Design review of the part built by this model. Coordinates are the model's own, in mm. A direction names the side the tool comes from. Give positions to 0.01 mm unless a question says otherwise; leave off trailing zeros. Write each loop counter-clockwise with the first axis right and the second up, starting at its lowest first coordinate (ties: lowest second). Pieces come first, ordered by that corner, then holes. Notation, with made-up numbers: (-34, 26) -> (3, 26) arc R32 ccw to (3, 63) -> close; hole circle Ø1 at (31, -17). An arc over 180 degrees is marked (long way). Answer as a JSON object with one key per item and string values.
```python
from build123d import *

# Parameters (mm, degrees)
F0_W     = 249.8
F0_H     = 100
F1_DEPTH = 4
F2_W     = 20
F2_H     = 10
F3_DEPTH = 25
F4_W     = 76
F4_H     = 40
F4_W_2   = 48
F4_H_2   = 65
F5_DEPTH = 25
F6_W     = 3.2
F6_H     = 20
F7_DEPTH = 13
F8_SIZE  = 12.1
F9_R     = 1


with BuildPart() as f1:
    # F0 (on Front) → F1 (new body)
    with BuildSketch(Plane.XZ):
        with Locations((45.308904, 9.584513)):
            Rectangle(F0_W, F0_H)
    extrude(amount=F1_DEPTH)

    # F2 (on face) → F3 (cut)
    with BuildSketch(Plane.XZ.offset(4)):
        with Locations((160.208904, -35.415487)):
            Rectangle(F2_W, F2_H)
        with Locations((-69.591096, -35.415487)):
            Rectangle(F2_W, F2_H)
    extrude(amount=-F3_DEPTH, mode=Mode.SUBTRACT)

    # F4 (on face) → F5 (cut)
    with BuildSketch(Plane.XZ.offset(4)):
        with Locations((45.308904, 21.584513)):
            Rectangle(F4_W, F4_H)
        with Locations((-55.591096, 27.084513)):
            Rectangle(F4_W_2, F4_H_2)
        with Locations((146.208904, 27.084513)):
            Rectangle(F4_W_2, F4_H_2)
    extrude(amount=-F5_DEPTH, mode=Mode.SUBTRACT)

    # F6 (on face) → F7 (join)
    with BuildSketch(Plane(origin=(0, 0, 0), x_dir=(-1, 0, 0), z_dir=(0, 1, 0))):
        with Locations((-123.808904, -17.415487)):
            Rectangle(F6_W, F6_H)
    extrude(amount=F7_DEPTH)

    # F8
    f8_edges = [f1.edges().sort_by_distance(p)[0] for p in [
        (123.808904, 13, -7.415487),
    ]]
    chamfer(f8_edges, length=F8_SIZE)

    # F9
    f9_edges = [f1.edges().sort_by_distance(p)[0] for p in [
        (123.808904, 13, -27.415487),
    ]]
    fillet(f9_edges, radius=F9_R)


solid = f1.part
```
(1) We need section B-B, the plane x = 29.5. State the section outline as (y, z) points.
Here are the results:
{"outline": "(-4, -40.42) -> (0, -40.42) -> (0, 1.58) -> (-4, 1.58) -> close; (-4, 41.58) -> (0, 41.58) -> (0, 59.58) -> (-4, 59.58) -> close"}
(2) We need section C-C, the plane x = -21. State the section outline as (y, z) points, then the cut area to 3 significant figures.
Here are the results:
{"outline": "(-4, -40.42) -> (0, -40.42) -> (0, 59.58) -> (-4, 59.58) -> close", "area": "400 mm²"}
(3) We need section A-A, the plane z = 11.5. State the section outline as (x, y) points, then the cut area to 3 significant figures.
Here are the results:
{"outline": "(-31.59, -4) -> (7.31, -4) -> (7.31, 0) -> (-31.59, 0) -> close; (83.31, -4) -> (122.21, -4) -> (122.21, 0) -> (83.31, 0) -> close", "area": "311 mm²"}
(4) For line 1 along Z through (x, y) = (40.5, -2); line 2 along X through (y, z) = (-0.75, 32); line 3 along Y through (x, z) = (102, -32.5), list the stretches that pass through material, from the lowest coordinate up.
Here are the results:
{"line 1": "z = -40.42 to 1.58, 41.58 to 59.58", "line 2": "x = -31.59 to 7.31, 83.31 to 122.21", "line 3": "y = -4 to 0"}
(5) We need section D-D, the plane z = 50.5. State the section outline as (x, y) points, then the cut area to 3 significant figures.
Here are the results:
{"outline": "(-31.59, -4) -> (122.21, -4) -> (122.21, 0) -> (-31.59, 0) -> close", "area": "615 mm²"}
(6) Clearance check with flat-ended pins moving along their axes: pin 1 (4.5 mm diameter, centred on y = -1.5, z = 27, fed in from -X); pin 2 (2.5 mm diameter, centred on x = 124.5, y = 7, fed in from -Z); pin 3 (4.5 mm diameter, centred on y = -2.5, z = -35, fed in from +X); pin 4 (3 mm diameter, centred on x = -7.5, y = 2.5, fed in from +Z). State where each tip first meets the part, or that it passes through.
Here are the results:
{"pin 1": "stops at x = -31.59", "pin 2": "stops at z = -27.42", "pin 3": "stops at x = 150.21", "pin 4": "passes through"}
(7) For faces 1 (the flat face through (122.209, 5, -20)), 2 (the flat face through (123.831, 7.035, -13.55)), 3 (the flat face through (125.409, 5, -20)), list the 3-axis set-ups (+Z, -Z, +X, -X, +Y, -Y) from which the entire face can be reached by the end or side of a thin tool; tool diameter is ignored.
Here are the results:
{"face 1": "+Z, -Z, -X, +Y", "face 2": "+Z, +X, -X, +Y", "face 3": "+Z, -Z, +X, +Y"}
